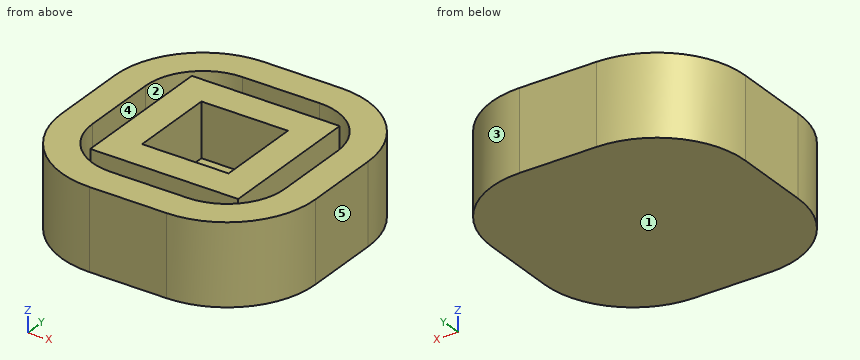
Autodesk Fusion 360 part; units mm, degrees
sketch "Boceto1" plane through (0, 0, 0) normal (0, 0, 1) x (1, 0, 0)
  line L0 (2, 5) -> (-2, 5)
  line L1 (-5, 2) -> (-5, -2)
  line L2 (-2, -5) -> (2, -5)
  line L3 (5, -2) -> (5, 2)
  line L4 (5, 5) -> (-5, -5) construction
  line L5 (-5, 5) -> (5, -5) construction
  line L6 (2.25, -2.25) -> (-2.25, -2.25)
  line L7 (-2.25, -2.25) -> (-2.25, 2.25)
  line L8 (-2.25, 2.25) -> (2.25, 2.25)
  line L9 (2.25, 2.25) -> (2.25, -2.25)
  line L10 (2.25, -2.25) -> (-2.25, 2.25) construction
  line L11 (-2.25, -2.25) -> (2.25, 2.25) construction
  line L12 (3.85, -3.85) -> (-3.85, -3.85)
  line L13 (-3.85, -3.85) -> (-3.85, 3.85)
  line L14 (-3.85, 3.85) -> (3.85, 3.85)
  line L15 (3.85, 3.85) -> (3.85, -3.85)
  arc A0 (-2, 5) -> (-5, 2) centre (-2, 2) ccw
  arc A1 (5, 2) -> (2, 5) centre (2, 2) ccw
  arc A2 (2, -5) -> (5, -2) centre (2, -2) ccw
  arc A3 (-5, -2) -> (-2, -5) centre (-2, -2) ccw
  arc A4 (-6.6, -2) -> (-2, -6.6) centre (-2, -2) ccw
  line L16 (-2, -6.6) -> (2, -6.6)
  arc A5 (2, -6.6) -> (6.6, -2) centre (2, -2) ccw
  line L17 (6.6, -2) -> (6.6, 2)
  arc A6 (6.6, 2) -> (2, 6.6) centre (2, 2) ccw
  line L18 (2, 6.6) -> (-2, 6.6)
  arc A7 (-2, 6.6) -> (-6.6, 2) centre (-2, 2) ccw
  line L19 (-6.6, 2) -> (-6.6, -2)
  dimension "d3" = 10
  dimension "d4" = 10
  dimension "d5" = 4.5
  dimension "d6" = 4.5
  dimension "d7" = -1.6
  dimension "d8" = 3
  dimension "d9" = 1.6
extrude "Extruir1" add sketch "Boceto1" along normal blind 1.4 contours L0 L1 L2 L3 A0 A1 A2 A3 | L6 L7 L8 L9 | L12 L13 L14 L15 | A4 L16 A5 L17 A6 L18 A7 L19
extrude "Extruir2" add sketch "Boceto1" along normal blind 2.8 from surface at 1.4 contours L12 L13 L14 L15
extrude "Extruir3" add sketch "Boceto1" along normal up to surface (2.8 mm away) from surface at 1.4 contours A4 L16 A5 L17 A6 L18 A7 L19
Verification items for the finished model (mm, model axes). Face numbers are marked on the shaded views. A direction names the side the tool comes from. Round coordinates to 2 decimals unless told otherwise and drop trailing zeros. Write each loop counter-clockwise with the first axis right and the second up, starting at its lowest first coordinate (ties: lowest second). Pieces come first, ordered by that corner, then holes. Notation, with made-up numbers: (67.5, 71.25) -> (100.5, 71.25) arc R21 ccw to (100.5, 80.25) -> close; hole circle Ø10 at (2.25, -12). An arc over 180 degrees is marked (long way). Write each question's results on one line, items separated by ' | '.
Q1. Sectioned sample at A-A, the plane z = 2.8. Record the boundary of the cut face in (x, y).
Derived:
outline: (-6.6, -2) arc R4.6 ccw to (-2, -6.6) -> (2, -6.6) arc R4.6 ccw to (6.6, -2) -> (6.6, 2) arc R4.6 ccw to (2, 6.6) -> (-2, 6.6) arc R4.6 ccw to (-6.6, 2) -> close; (-3.85, -3.85) -> (3.85, -3.85) -> (3.85, 3.85) -> (-3.85, 3.85) -> close; hole (-5, -2) arc R3 ccw to (-2, -5) -> (2, -5) arc R3 ccw to (5, -2) -> (5, 2) arc R3 ccw to (2, 5) -> (-2, 5) arc R3 ccw to (-5, 2) -> close; hole (-2.25, -2.25) -> (2.25, -2.25) -> (2.25, 2.25) -> (-2.25, 2.25) -> close
Q2. Access from +Z, -Z, +X, -X, +Y, -Y to the whole of each face (thin tool, end or side, straight path). Record for the marked faces 1 and 2.
Derived:
face 1: -Z, +X, -X, +Y, -Y | face 2: +Z
Q3. Sectioned sample at B-B, the plane y = 0.25. Record the boundary of the cut face in (x, z), and give its area (3 significant figures).
Derived:
outline: (-6.6, 0) -> (6.6, 0) -> (6.6, 4.2) -> (5, 4.2) -> (5, 1.4) -> (3.85, 1.4) -> (3.85, 4.2) -> (2.25, 4.2) -> (2.25, 1.4) -> (-2.25, 1.4) -> (-2.25, 4.2) -> (-3.85, 4.2) -> (-3.85, 1.4) -> (-5, 1.4) -> (-5, 4.2) -> (-6.6, 4.2) -> close | area: 36.4 mm²
Q4. Sectioned sample at D-D, the plane x = -2.75. Record the boundary of the cut face in (y, z).
Derived:
outline: (-6.54, 0) -> (6.54, 0) -> (6.54, 4.2) -> (4.9, 4.2) -> (4.9, 1.4) -> (3.85, 1.4) -> (3.85, 4.2) -> (-3.85, 4.2) -> (-3.85, 1.4) -> (-4.9, 1.4) -> (-4.9, 4.2) -> (-6.54, 4.2) -> close
Q5. Go/stop test with flat-tipped pins: pin 1 Ø2 at (x, z) = (-3, 0.5) entering from +Y; pin 2 Ø1.5 at (y, z) = (-5, 2.5) entering from +X. Record where each tip stops, or that it passes through.
Derived:
pin 1: stops at y = 6.6 | pin 2: stops at x = 6.01
Q6. Draft check along Y on the marked faces 3, 4 and 5. Enter one of: released by +Y, released by -Y, zero draft, split by the parting line, or undercut.
Derived:
face 3: released by +Y | face 4: undercut | face 5: zero draft
Q7. Thickness scan on probe 1 along X at (y, z) = (-0.25, 2.55); probe 2 along Z at (x, y) = (2, 0.5). Record the ranges inside material, lowest first.
Derived:
probe 1: x = -6.6 to -5, -3.85 to -2.25, 2.25 to 3.85, 5 to 6.6 | probe 2: z = 0 to 1.4
